The model under review builds one solid part; all positions refer to its coordinate system, in mm. Face numbers are marked on the shaded views. A direction names the side the tool comes from. Round coordinates to 2 decimals unless told otherwise and drop trailing zeros. Order: outer loops, then holes, each group sorted by start corner. A loop starts at its lowest first (then second) coordinate and runs counter-clockwise, first axis right, second up. Notation, with made-up numbers: M 53.25,48 L 64.25,48 A26 ccw 64.25,83 Z; hole C 49.5,-1 d9. An arc over 180 degrees is marked long. Use a Markdown table: item, result. Add a question column.
1. For the marked faces 1, 2 and 3, list the 3-axis set-ups (+Z, -Z, +X, -X, +Y, -Y) from which the entire face can be reached by the end or side of a thin tool; tool diameter is ignored.
2. Consider section A-A on x = 35. State the section outline as (y, z) points, then the cut area to 3 significant figures.
3. Consider section B-B on y = 0. State the section outline as (x, z) points.
4. To check wall thickness, follow probe 1 along Z at (x, y) = (-12, -16.5); probe 2 along Z at (x, y) = (-38.5, -9); probe 3 along Y at (x, z) = (-14.5, 41.5). State the ranges of each line that lie inside material, in increasing order.
5. Consider section D-D on z = -13. State the section outline as (x, y) points, then the cut area to 3 significant figures.
6. The part is to be moulded in two halves that separate along Y. For the marked faces 4, 5 and 6, say which applies: +Y half, -Y half, draft (parallel to the pull), parting line (faces both ways), or undercut.
7. Consider section C-C on z = 35. State the section outline as (x, y) points.
8. Insertion check: P1, Ø1.5, axis at x = 29.5, y = 37.5, coming from the +Z side; P2, Ø9, axis at x = -5.5, z = 35.5, coming from the -Y side; P3, Ø12, axis at x = -24, y = 0, coming from the -Z side. Each pin has a flat end and moves straight along its axis. Give the tip position at first contact, or say it passes through.
from build123d import *

# Parameters (mm, degrees)
F0_W     = 100
F0_H     = 10
F1_DEPTH = 50
F2_R     = 12.5
F3_DEPTH = 15
F4_R     = 10
F5_R     = 25
F5_W     = 30
F5_H     = 30
F6_DEPTH = 50


with BuildPart() as f1:
    # F0 (on Front) → F1 (new body, symmetric)
    with BuildSketch(Plane.XZ):
        Rectangle(F0_W, F0_H)
    extrude(amount=F1_DEPTH, both=True)

    # F2 (on face) → F3 (join)
    with BuildSketch(Plane(origin=(0, 0, -5), x_dir=(1, 0, 0), z_dir=(0, 0, -1))):
        with Locations((35, 35)):
            Circle(F2_R)
        with Locations((35, -35)):
            Circle(F2_R)
        with Locations((-35, -35)):
            Circle(F2_R)
        with Locations((-35, 35)):
            Circle(F2_R)
    extrude(amount=F3_DEPTH)

    # F4
    f4_edges = [f1.edges().sort_by_distance(p)[0] for p in [
        (-50, -50, 0),
        (50, -50, 0),
        (50, 50, 0),
        (-50, 50, 0),
    ]]
    fillet(f4_edges, radius=F4_R)

    # F5 (on face) → F6 (join)
    with BuildSketch(Plane.XY.offset(5)):
        Circle(F5_R)
        Rectangle(F5_W, F5_H, mode=Mode.SUBTRACT)
    extrude(amount=F6_DEPTH)


solid = f1.part
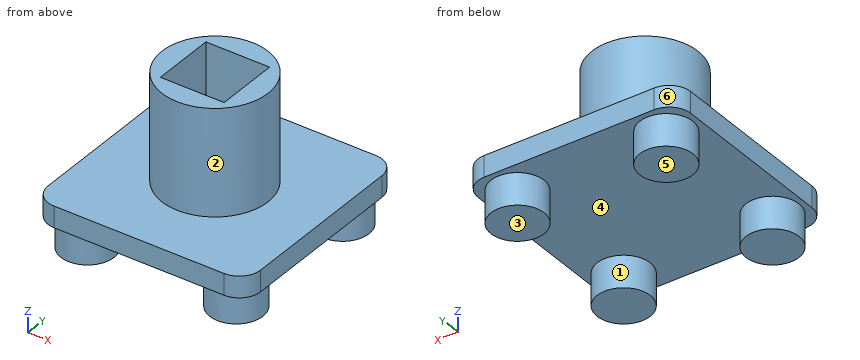
Answer block:
| question | item | result |
|---|---|---|
| 1 | face 1 | -Z |
| 1 | face 2 | +Z |
| 1 | face 3 | -Z, +X, -X, +Y, -Y |
| 2 | outline | M -50,-5 L -47.5,-5 L -47.5,-20 L -22.5,-20 L -22.5,-5 L 22.5,-5 L 22.5,-20 L 47.5,-20 L 47.5,-5 L 50,-5 L 50,5 L -50,5 Z |
| 2 | area | 1,750 mm^2 |
| 3 | outline | M -50,-5 L 50,-5 L 50,5 L 25,5 L 25,55 L 15,55 L 15,5 L -15,5 L -15,55 L -25,55 L -25,5 L -50,5 Z |
| 4 | probe 1 | -5 to 55 |
| 4 | probe 2 | -5 to 5 |
| 4 | probe 3 | -20.37 to -15, 15 to 20.37 |
| 5 | outline | C -35,-35 d25; C -35,35 d25; C 35,-35 d25; C 35,35 d25 |
| 5 | area | 1,960 mm^2 |
| 6 | face 4 | undercut |
| 6 | face 5 | draft |
| 6 | face 6 | +Y half |
| 7 | outline | C 0,0 d50; hole M -15,-15 L 15,-15 L 15,15 L -15,15 Z |
| 8 | P1 | z = 5 |
| 8 | P2 | y = -24.98 |
| 8 | P3 | z = -5 |
